Verification items for the finished model (mm, model axes). Coordinates: 2 decimals unless noted, no trailing zeros. Order: outer loops, then holes, each group sorted by start corner. A loop starts at its lowest first (then second) coordinate and runs counter-clockwise, first axis right, second up. Notation, with made-up numbers: (66.5, 87.5) -> (117.5, 87.5) arc R32 cw to (117.5, 119.5) -> close; hole circle Ø1 at (0.5, 68). An arc over 180 degrees is marked (long way). Write item = value, one per line. Start each with the question number.
1. Cross-section at A-A on x = 1.8. Record the cut outline in (y, z).
2. Thickness scan on line 1 along Y through (x, z) = (3.65, -21.5); line 2 along Y through (x, z) = (0.8, -22.5); line 3 along Z through (x, y) = (1.1, -16). Record the ranges inside material, lowest first. Write a range as from..to.
3. Cross-section at D-D on z = -2.5. Record the cut outline in (x, y), plus the area to 3 significant figures.
4. Cross-section at B-B on y = -12. Record the cut outline in (x, z).
5. Go/stop test with flat-tipped pins: P1, Ø3.5, axis at y = -3, z = -3, coming from the +X side; P2, Ø1.5, axis at x = 1, z = -5, coming from the -Y side; P3, Ø2, axis at x = 2, z = -11, coming from the -Y side. Record where each tip stops, or that it passes through.
6. Release check for a two-part mould opening along Z. For faces 1 (the cylindrical face through (1.972, -13.505, -14.048)), 2 (the flat face through (1.97, -22.75, -32.03)), 3 (the flat face through (2, -10, 0)) record: +Z half, -Z half, draft (parallel to the pull), parting line (faces both ways), or undercut.
7. Cross-section at C-C on z = -20. Record the cut outline in (x, y).
from build123d import *

# Parameters (mm, degrees)
SKETCH1_R           = 1.3
BOSS_EXTRUDE1_DEPTH = 4
SKETCH2_R           = 9.15
CUT_EXTRUDE1_DEPTH  = 52.522207254
FILLET1_R           = 4


with BuildPart() as part:
    # Sketch1 → Boss-Extrude1 (new body)
    with BuildSketch(Plane(origin=(0, 0, 0), x_dir=(0, 0, -1), z_dir=(1, 0, 0))):
        Polygon((45, 0), (22.5, 4.769696007), (0, 0), (0, -20), (22.5, -24.769696007), (45, -20), align=None)
        with Locations((22.5, 0.680807118)):
            Circle(SKETCH1_R, mode=Mode.SUBTRACT)
        with Locations((22.5, -20.680807118)):
            Circle(SKETCH1_R, mode=Mode.SUBTRACT)
        with Locations((42, -3)):
            Circle(SKETCH1_R, mode=Mode.SUBTRACT)
        with Locations((3, -3)):
            Circle(SKETCH1_R, mode=Mode.SUBTRACT)
        with Locations((3, -17)):
            Circle(SKETCH1_R, mode=Mode.SUBTRACT)
        with Locations((42, -17)):
            Circle(SKETCH1_R, mode=Mode.SUBTRACT)
    extrude(amount=BOSS_EXTRUDE1_DEPTH)

    # Sketch2 → Cut-Extrude1 (cut, through all)
    with BuildSketch(Plane.ZY):
        with Locations((-22.5, -10)):
            Circle(SKETCH2_R)
    extrude(amount=-CUT_EXTRUDE1_DEPTH, mode=Mode.SUBTRACT)

    # Fillet1
    fillet1_edges = [part.edges().sort_by_distance(p)[0] for p in [
        (2, -20, 0),
        (2, 0, 0),
        (2, 0, -45),
        (2, -20, -45),
    ]]
    fillet(fillet1_edges, radius=FILLET1_R)


solid = part.part
Worked out:
q1.outline = (-24.77, -22.5) -> (-20.67, -41.83) arc R4 ccw to (-16.76, -45) -> (-3.24, -45) arc R4 ccw to (0.67, -41.83) -> (4.77, -22.5) -> (0.67, -3.17) arc R4 ccw to (-3.24, 0) -> (-16.76, 0) arc R4 ccw to (-20.67, -3.17) -> close; hole circle Ø2.6 at (-20.68, -22.5); hole circle Ø18.3 at (-10, -22.5); hole circle Ø2.6 at (-17, -42); hole circle Ø2.6 at (-17, -3); hole circle Ø2.6 at (-3, -42); hole circle Ø2.6 at (-3, -3); hole circle Ø2.6 at (0.68, -22.5)
q2.line_1 = -24.56..-21.51, -19.85..-19.1, -0.9..-0.15, 1.51..4.56
q2.line_2 = -24.77..-21.98, -19.38..-19.15, -0.85..-0.62, 1.98..4.77
q2.line_3 = -45..-42.83, -41.17..-29.41, -15.59..-3.83, -2.17..0
q3.outline = (0, -20.47) -> (4, -20.47) -> (4, -18.2) -> (0, -18.2) -> close; (0, -15.8) -> (4, -15.8) -> (4, -4.2) -> (0, -4.2) -> close; (0, -1.8) -> (4, -1.8) -> (4, 0.47) -> (0, 0.47) -> close
q3.area = 64.5 mm²
q4.outline = (0, -45) -> (4, -45) -> (4, -31.43) -> (0, -31.43) -> close; (0, -13.57) -> (4, -13.57) -> (4, 0) -> (0, 0) -> close
q5.P1 = 4
q5.P2 = -21.22
q5.P3 = -22.54
q6.face_1 = undercut
q6.face_2 = -Z half
q6.face_3 = +Z half
q7.outline = (0, -24.24) -> (4, -24.24) -> (4, -18.8) -> (0, -18.8) -> close; (0, -1.2) -> (4, -1.2) -> (4, 4.24) -> (0, 4.24) -> close
